from build123d import *

# Parameters (mm, degrees)
BOSS_EXTRUDE1_DEPTH = 12.7
SKETCH2_R           = 9.525
CUT_EXTRUDE1_DEPTH  = 218.403821494
SKETCH3_W           = 76.2
SKETCH3_H           = 6.35
SKETCH3_W_2         = 12.7
SKETCH3_H_2         = 25.4
BOSS_EXTRUDE2_DEPTH = 12.7
SKETCH9_R           = 22.225
CUT_EXTRUDE4_DEPTH  = 218.403821494
CUT_EXTRUDE6_DEPTH  = 218.403821494
BOSS_EXTRUDE3_DEPTH = 12.7
SKETCH15_R          = 1.27
CUT_EXTRUDE8_DEPTH  = 218.403821494
SKETCH13_R          = 3.126994
SKETCH13_W          = 19.05
SKETCH13_H          = 36.998088235
CUT_EXTRUDE9_DEPTH  = 218.403821494
FILLET1_R           = 2.54
FILLET2_R           = 2.54


with BuildPart() as part:
    # Sketch1 → Boss-Extrude1 (new body)
    with BuildSketch(Plane(origin=(0, 0, 0), x_dir=(0, 0, -1), z_dir=(1, 0, 0))):
        with BuildLine():
            ThreePointArc((57.15, 81.28), (21.180615335, 49.546911859), (-25.4, 38.1))
            Line((-25.4, 38.1), (-76.2, 38.1))
            Line((-76.2, 38.1), (-76.2, 44.45))
            Line((-76.2, 44.45), (-127, 44.45))
            Line((-127, 44.45), (-127, 38.1))
            Line((-127, 38.1), (-165.1, 38.1))
            Line((-165.1, 38.1), (-165.1, -38.1))
            Line((-165.1, -38.1), (177.8, -38.1))
            Line((177.8, -38.1), (139.7, 38.1))
            Line((139.7, 38.1), (139.7, 124.46))
            ThreePointArc((139.7, 124.46), (93.119384665, 113.013088141), (57.15, 81.28))
        make_face()
    extrude(amount=BOSS_EXTRUDE1_DEPTH)

    # Sketch2 → Cut-Extrude1 (cut, through all)
    with BuildSketch(Plane(origin=(12.7, 0, 0), x_dir=(0, 0, -1), z_dir=(1, 0, 0))):
        with Locations((111.125, 82.55)):
            Circle(SKETCH2_R)
    extrude(amount=-CUT_EXTRUDE1_DEPTH, mode=Mode.SUBTRACT)

    # Sketch3 → Boss-Extrude2 (add)
    with BuildSketch(Plane(origin=(12.7, 0, 0), x_dir=(0, 0, -1), z_dir=(1, 0, 0))):
        with Locations((114.3, -41.275)):
            Rectangle(SKETCH3_W, SKETCH3_H)
        with Locations((-63.5, -41.275)):
            Rectangle(SKETCH3_W, SKETCH3_H)
        with Locations((-171.45, 0)):
            Rectangle(SKETCH3_W_2, SKETCH3_H_2)
    extrude(amount=-BOSS_EXTRUDE2_DEPTH)

    # Sketch9 → Cut-Extrude4 (cut, through all)
    with BuildSketch(Plane(origin=(12.7, 0, 0), x_dir=(0, 0, -1), z_dir=(1, 0, 0))):
        with Locations((-19.05, 0)):
            Circle(SKETCH9_R)
    extrude(amount=-CUT_EXTRUDE4_DEPTH, mode=Mode.SUBTRACT)

    # Sketch12 → Cut-Extrude6 (cut, through all)
    with BuildSketch(Plane(origin=(12.7, 0, 0), x_dir=(0, 0, -1), z_dir=(1, 0, 0))):
        Polygon((139.7, 9.701936686), (139.7, -25.4), (157.250968343, -25.4), align=None)
        Polygon((109.05604179, 15.875), (127, -13.283932092), (127, 45.033932092), align=None)
        Polygon((119.54395821, -25.4), (101.6, 3.758932092), (83.65604179, -25.4), align=None)
        Polygon((76.2, -13.283932092), (94.14395821, 15.875), (76.2, 45.033932092), align=None)
        Polygon((-57.15, -18.203333333), (-57.15, 18.203333333), (-91.28125, 0), align=None)
        Polygon((-70.64375, -25.4), (-104.775, -7.196666667), (-138.90625, -25.4), align=None)
        Polygon((-152.4, -18.203333333), (-118.26875, 0), (-152.4, 18.203333333), align=None)
        Polygon((-104.775, 7.196666667), (-70.64375, 25.4), (-138.90625, 25.4), align=None)
    extrude(amount=-CUT_EXTRUDE6_DEPTH, mode=Mode.SUBTRACT)

    # Sketch14 → Boss-Extrude3 (add)
    with BuildSketch(Plane(origin=(12.7, 0, 0), x_dir=(0, 0, -1), z_dir=(1, 0, 0))):
        Polygon((147.390774674, 22.718450651), (170.109225326, -22.718450651), (175.788837989, -19.87864432), (153.070387337, 25.558256983), align=None)
    extrude(amount=-BOSS_EXTRUDE3_DEPTH)

    # Sketch15 → Cut-Extrude8 (cut, through all)
    with BuildSketch(Plane(origin=(12.7, 0, 0), x_dir=(0, 0, -1), z_dir=(1, 0, 0))):
        with Locations((-166.14759319, -13.417947427)):
            Circle(SKETCH15_R)
        with Locations((-127.867535363, 39.027514093)):
            Circle(SKETCH15_R)
        with Locations((-102.468735692, -39.026389927)):
            Circle(SKETCH15_R)
        with Locations((75.20280066, -38.886443562)):
            Circle(SKETCH15_R)
        with Locations((153.276127819, -39.019402004)):
            Circle(SKETCH15_R)
        with Locations((-24.501616142, -38.997667224)):
            Circle(SKETCH15_R)
        with Locations((-166.09635678, 13.487510741)):
            Circle(SKETCH15_R)
        with Locations((-75.205348286, 38.8896632)):
            Circle(SKETCH15_R)
        with Locations((171.314053114, -23.120059914)):
            Circle(SKETCH15_R)
        with Locations((147.792383937, 23.92327844)):
            Circle(SKETCH15_R)
    extrude(amount=-CUT_EXTRUDE8_DEPTH, mode=Mode.SUBTRACT)

    # Sketch13 → Cut-Extrude9 (cut, through all)
    with BuildSketch(Plane(origin=(12.7, 0, 0), x_dir=(0, 0, -1), z_dir=(1, 0, 0))):
        with Locations((44.45, -25.4)):
            Circle(SKETCH13_R)
        with Locations((57.15, -25.4)):
            Circle(SKETCH13_R)
        with Locations((44.45, -12.7)):
            Circle(SKETCH13_R)
        with Locations((57.15, -12.7)):
            Circle(SKETCH13_R)
        with Locations((44.45, 0)):
            Circle(SKETCH13_R)
        with Locations((57.15, 0)):
            Circle(SKETCH13_R)
        with Locations((53.975, 31.199044118)):
            Rectangle(SKETCH13_W, SKETCH13_H)
        Polygon((31.75, -25.4), (31.75, 38.736971741), (0.2156773, -25.4), align=None)
    extrude(amount=-CUT_EXTRUDE9_DEPTH, mode=Mode.SUBTRACT)

    # Fillet1
    fillet1_edges = [part.edges().sort_by_distance(p)[0] for p in [
        (6.35, -25.4, -139.7),
        (6.35, 9.701936686, -139.7),
        (6.35, -25.4, -157.250968343),
        (6.35, 0, 118.26875),
        (6.35, -18.203333333, 152.4),
        (6.35, 18.203333333, 152.4),
        (6.35, -25.4, 70.64375),
        (6.35, -25.4, 138.90625),
        (6.35, -7.196666667, 104.775),
        (6.35, 7.196666667, 104.775),
        (6.35, 25.4, 138.90625),
        (6.35, 25.4, 70.64375),
        (6.35, 3.758932092, -101.6),
        (6.35, -25.4, -119.54395821),
        (6.35, -25.4, -83.65604179),
        (6.35, 45.033932092, -127),
        (6.35, -13.283932092, -127),
        (6.35, 15.875, -109.05604179),
        (6.35, 15.875, -94.14395821),
        (6.35, -13.283932092, -76.2),
        (6.35, 45.033932092, -76.2),
        (6.35, 18.203333333, 57.15),
        (6.35, -18.203333333, 57.15),
        (6.35, 0, 91.28125),
    ]]
    fillet(fillet1_edges, radius=FILLET1_R)

    # Fillet2
    fillet2_edges = [part.edges().sort_by_distance(p)[0] for p in [
        (6.35, -25.4, -31.75),
        (6.35, -25.4, -0.2156773),
        (6.35, 38.736971741, -31.75),
        (6.35, 49.698088235, -63.5),
        (6.35, 12.7, -63.5),
        (6.35, 12.7, -44.45),
        (6.35, 49.698088235, -44.45),
    ]]
    fillet(fillet2_edges, radius=FILLET2_R)


solid = part.part
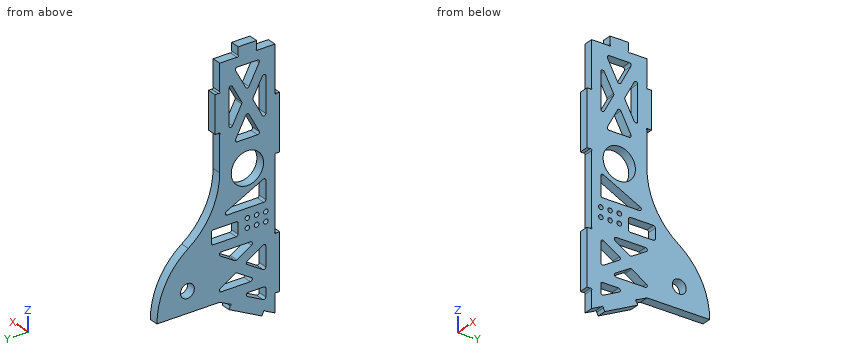
Verification items for the finished model (mm, model axes). Coordinates: 2 decimals unless noted, no trailing zeros. Order: outer loops, then holes, each group sorted by start corner. A loop starts at its lowest first (then second) coordinate and runs counter-clockwise, first axis right, second up. Notation, with made-up numbers: (-7.5, 36) -> (43.5, 36) arc R15 cw to (43.5, 58) -> close; hole circle Ø1 at (40, -21.5). An arc over 180 degrees is marked (long way). Put each result on its own line as item: value. Start each with the question number.
1. Cross-section at C-C, the plane x = 5.75. Count the separate pieces of the cut face and the enclosed holes in it, then the cut area to 3 significant figures.
2. Material ranges on L1, parallel to Y at x = 10.25, z = -57.15; L2, parallel to Z at x = 0.75, y = 37.5; L3, parallel to Y at x = 11.5, z = 79.5, recorded low to high. Write a range as [from, to].
3. Go/stop test with flat-tipped pins: pin 1 Ø15 at (y, z) = (82.55, -111.125) entering from +X; pin 2 Ø1.5 at (x, z) = (8.5, 110.5) entering from +Y; pin 3 Ø4 at (x, z) = (3.5, -51.5) entering from +Y; pin 4 Ø3.5 at (x, y) = (7, -42.5) entering from -Z. Record where each tip stops, or that it passes through.
4. Cross-section at D-D, the plane y = 57. Record the boundary of the cut face in (x, z), then the cut area to 3 significant figures.
5. Cross-section at A-A, the plane z = -16. Record the boundary of the cut face in (x, y).
6. Cross-section at B-B, the plane y = 88.5. Record the boundary of the cut face in (x, z), then the cut area to 3 significant figures.
Computed:
1. separate pieces: 1
1. enclosed holes: 18
1. area: 25,900 mm2
2. L1: [-38.1, -28.53], [-22.27, -15.83], [-9.57, -3.13], [3.13, 12.7], [49.7, 81.28]
2. L2: [-140, -126.55], [-122.37, -80.83], [-76.65, -63.5], [-44.45, 165.1]
2. L3: [-44.45, -25.04], [-20.68, -6.28], [6.28, 20.68], [25.04, 44.45]
3. pin 1: through
3. pin 2: y = 44.45
3. pin 3: y = 76.35
3. pin 4: z = -152.4
4. outline: (0, -139.7) -> (12.7, -139.7) -> (12.7, -33.27) -> (0, -33.27) -> close
4. area: 1,350 mm2
5. outline: (0, -38.1) -> (12.7, -38.1) -> (12.7, -25.4) -> (0, -25.4) -> close; (0, 6.7) -> (12.7, 6.7) -> (12.7, 47.02) -> (0, 47.02) -> close
6. outline: (0, -139.7) -> (12.7, -139.7) -> (12.7, -118.56) -> (0, -118.56) -> close; (0, -103.69) -> (12.7, -103.69) -> (12.7, -62.66) -> (0, -62.66) -> close
6. area: 789 mm2
